```python
from build123d import *

# Parameters (mm, degrees)
F0_W     = 42.8625
F0_H     = 42.8625
F0_R     = 10.31875
F1_DEPTH = 42.8625
F2_R     = 10.31875
F3_DEPTH = 42.8635
F4_R     = 0.508
F5_R     = 0.508
F6_R     = 0.508


with BuildPart() as f1:
    # F0 (on Front) → F1 (new body)
    with BuildSketch(Plane.XZ):
        Rectangle(F0_W, F0_H)
        Circle(F0_R, mode=Mode.SUBTRACT)
    extrude(amount=F1_DEPTH)

    # F2 (on face) → F3 (cut, through all)
    with BuildSketch(Plane.XY.offset(21.43125)):
        with Locations((0, -21.43125)):
            Circle(F2_R)
    extrude(amount=-F3_DEPTH, mode=Mode.SUBTRACT)

    # F4
    f4_edges = [f1.edges().sort_by_distance(p)[0] for p in [
        (0, -42.8625, 21.43125),
    ]]
    fillet(f4_edges, radius=F4_R)

    # F5
    f5_edges = [f1.edges().sort_by_distance(p)[0] for p in [
        (21.43125, -21.17725, 21.43125),
        (21.43125, 0, 0),
        (21.43125, -21.43125, -21.43125),
        (-21.43125, -42.8625, -0.254),
        (0, -42.8625, -21.43125),
        (0, 0, -21.43125),
        (-21.43125, -21.43125, -21.43125),
        (0, 0, 21.43125),
        (21.43125, -42.8625, -0.254),
        (0, -42.8625, 20.92325),
        (-21.43125, 0, 0),
        (-21.43125, -21.17725, 21.43125),
    ]]
    fillet(f5_edges, radius=F5_R)

    # F6
    f6_edges = [f1.edges().sort_by_distance(p)[0] for p in [
        (-10.31875, -42.8625, 0),
        (-10.31875, -21.43125, -21.43125),
        (-10.31875, -21.43125, 21.43125),
        (-10.31875, 0, 0),
    ]]
    fillet(f6_edges, radius=F6_R)


solid = f1.part
```
Geometry check sheet. Reference: the model listing, model coordinates, mm. Give positions to 0.01 mm unless a question says otherwise; leave off trailing zeros. Loops run counter-clockwise (first coordinate to the right, second up) from the corner with the lowest first, then second, coordinate; pieces in that order, holes last. Notation, with made-up numbers: M 6.5,29 L 43.5,29 A32 cw 43.5,55 Z; hole C 16,-16 d10. An arc over 180 degrees is marked long. Write item = value, one per line.
(1) Gauge pin test, flat end, axial feed: pin 1 Ø2 at (x, y) = (-5.5, -13.5) entering from +Z. Record the tip position at first contact, or that the pin passes through.
Answer below:
pin_1 = 21.4
(2) Sectioned sample at C-C, the plane x = -8. State how many separate pieces and enclosed holes the cut face has, plus the area to 3 significant figures.
Answer below:
separate_pieces = 4
enclosed_holes = 0
area = 889 mm2
(3) Sectioned sample at B-B, the plane y = -9. Record the cut outline in (x, z), plus the area to 3 significant figures.
Answer below:
outline = M -21.43,-20.92 A0.51 ccw -20.92,-21.43 L 20.92,-21.43 A0.51 ccw 21.43,-20.92 L 21.43,20.92 A0.51 ccw 20.92,21.43 L -20.92,21.43 A0.51 ccw -21.43,20.92 Z; hole C 0,0 d20.64
area = 1,500 mm2
(4) Sectioned sample at A-A, the plane x = 0. Record the cut outline in (y, z), plus the area to 3 significant figures.
Answer below:
outline = M -42.86,-20.92 A0.51 ccw -42.35,-21.43 L -32.26,-21.43 A0.51 ccw -31.75,-20.92 L -31.75,-10.32 L -42.35,-10.32 A0.51 ccw -42.86,-10.83 Z; M -42.86,10.83 A0.51 ccw -42.35,10.32 L -31.75,10.32 L -31.75,20.92 A0.51 ccw -32.26,21.43 L -42.35,21.43 A0.51 ccw -42.86,20.92 Z; M -11.11,-20.92 A0.51 ccw -10.6,-21.43 L -0.51,-21.43 A0.51 ccw 0,-20.92 L 0,-10.83 A0.51 ccw -0.51,-10.32 L -11.11,-10.32 Z; M -11.11,10.32 L -0.51,10.32 A0.51 ccw 0,10.83 L 0,20.92 A0.51 ccw -0.51,21.43 L -10.6,21.43 A0.51 ccw -11.11,20.92 Z
area = 493 mm2
(5) Material ranges on line 1 (X direction, y = -10.5, z = 0); line 2 (Y direction, x = 0, z = 16); line 3 (X direction, y = -26, z = -12.5), recorded low to high. Write a range as [from, to].
Answer below:
line_1 = [-21.43, -10.32], [10.32, 21.43]
line_2 = [-42.86, -31.75], [-11.11, 0]
line_3 = [-21.43, -9.25], [9.25, 21.43]
(6) Release check for a two-part mould opening along Y. For faces 1 (the face through (-7.61, -14.46, -12.64)), 2 (the face through (-10, -30, -21.431)), 3 (the face through (-10, -42.862, -9)) record: released by +Y, released by -Y, zero draft, split by the parting line, or undercut.
Answer below:
face_1 = undercut
face_2 = zero draft
face_3 = released by -Y
